```python
from build123d import *

# Parameters (mm, degrees)
F1_DEPTH = 63.5
F2_DEPTH = 63.5
F3_R     = 2.440759
F3_R_2   = 3.868434
F3_R_3   = 2.279206
F4_DEPTH = 25.4


with BuildPart() as f1:
    # F0 (on Right) → F1 (new body)
    with BuildSketch(Plane.YZ):
        Polygon((0, 0), (-51.902805, 0), (-51.902805, -8.131986), (-6.712981, -8.131986), (-6.712981, -66.856928), (0, -66.856928), align=None)
    extrude(amount=F1_DEPTH)

    # F1_face (on face) → F2 (join)
    with BuildSketch(Plane(origin=(0, -15.039437, -20.209903), x_dir=(0, 1, 0), z_dir=(-1, 0, 0))):
        Polygon((-36.863367, -20.209903), (15.039437, -20.209903), (15.039437, 46.647025), (8.326457, 46.647025), (8.326457, -12.077918), (-36.863367, -12.077918), align=None)
    extrude(amount=F2_DEPTH)

    # F3 (on face) → F4 (cut)
    with BuildSketch(Plane.XZ.offset(6.712981)):
        with Locations((-52.33942, -15.991084)):
            Circle(F3_R)
        with Locations((-42.733856, -16.209394)):
            Circle(F3_R_2)
        with Locations((-32.691672, -16.864318)):
            Circle(F3_R_3)
        with Locations((32.691672, -16.864318)):
            Circle(F3_R_3)
        with Locations((42.733856, -16.209394)):
            Circle(F3_R_2)
        with Locations((52.33942, -15.991084)):
            Circle(F3_R)
        with Locations((52.33942, -58.997829)):
            Circle(F3_R)
        with Locations((42.733856, -58.77952)):
            Circle(F3_R_2)
        with Locations((32.691672, -58.124595)):
            Circle(F3_R_3)
        with Locations((-52.33942, -58.997829)):
            Circle(F3_R)
        with Locations((-42.733856, -58.77952)):
            Circle(F3_R_2)
        with Locations((-32.691672, -58.124595)):
            Circle(F3_R_3)
    extrude(amount=-F4_DEPTH, mode=Mode.SUBTRACT)


solid = f1.part
```
Can you work these out from the model? Positions are in its coordinate system, mm. A direction names the side the tool comes from. Round coordinates to 2 decimals unless told otherwise and drop trailing zeros. Order: outer loops, then holes, each group sorted by start corner. A loop starts at its lowest first (then second) coordinate and runs counter-clockwise, first axis right, second up. Notation, with made-up numbers: (56, 24) -> (76, 24) arc R7 cw to (76, 31) -> close; hole circle Ø8 at (84.25, -13.75). An arc over 180 degrees is marked (long way). Return JSON: item names as keys, results as strings. Group by question number.
1. I need wall thicknesses on line 1 (Z direction, x = 20, y = -17.5); line 2 (Y direction, x = 8, z = -32). Which ranges of each line are inside material? Lowest first, please. Write a range as [from, to].
2. If we section it at A-A, the plane x = 43: Write out the boundary of the cut face in (y, z).
3. Will these pins go through, and if not, where does the flat tip stop? pin 1 (17.5 mm diameter, centred on x = 26.5, z = -44.5, fed in from -Y); pin 2 (8 mm diameter, centred on x = 45, y = -28, fed in from -Z).
4. Which directions (+Z, -Z, +X, -X, +Y, -Y) give clear straight access to the entire face, cutting with the end or side of a thin tool? Please do faces 1 (the face through (54.594, -3.403, -59.933)), 2 (the face through (-31, -29, -8.132)).
5. We'd pull the mould along X, two halves only. Please class faces 3 (the face through (54.594, -3.403, -16.926)), 4 (the face through (-31, -6.713, -38)), 5 (the face through (-33.19, -3.4, -60.35)): released by +X, released by -X, zero draft, split by the parting line, or undercut.
6. If we section it at C-C, the plane y = -5: Count the separate pieces of the cut face and the enclosed holes in it, then the cut area to 3 significant figures.
Output values:
{
 "1": {"line 1": "[-8.13, 0]", "line 2": "[-6.71, 0]"},
 "2": {"outline": "(-51.9, -8.13) -> (-6.71, -8.13) -> (-6.71, -12.35) -> (0, -12.35) -> (0, 0) -> (-51.9, 0) -> close; (-6.71, -66.86) -> (0, -66.86) -> (0, -62.64) -> (-6.71, -62.64) -> close; (-6.71, -54.92) -> (0, -54.92) -> (0, -20.07) -> (-6.71, -20.07) -> close"},
 "3": {"pin 1": "y = -6.71", "pin 2": "z = -8.13"},
 "4": {"face 1": "+Y, -Y", "face 2": "-Z, +X, -X, -Y"},
 "5": {"face 3": "undercut", "face 4": "zero draft", "face 5": "undercut"},
 "6": {"separate pieces": "1", "enclosed holes": "12", "area": "8,160 mm²"}
}
